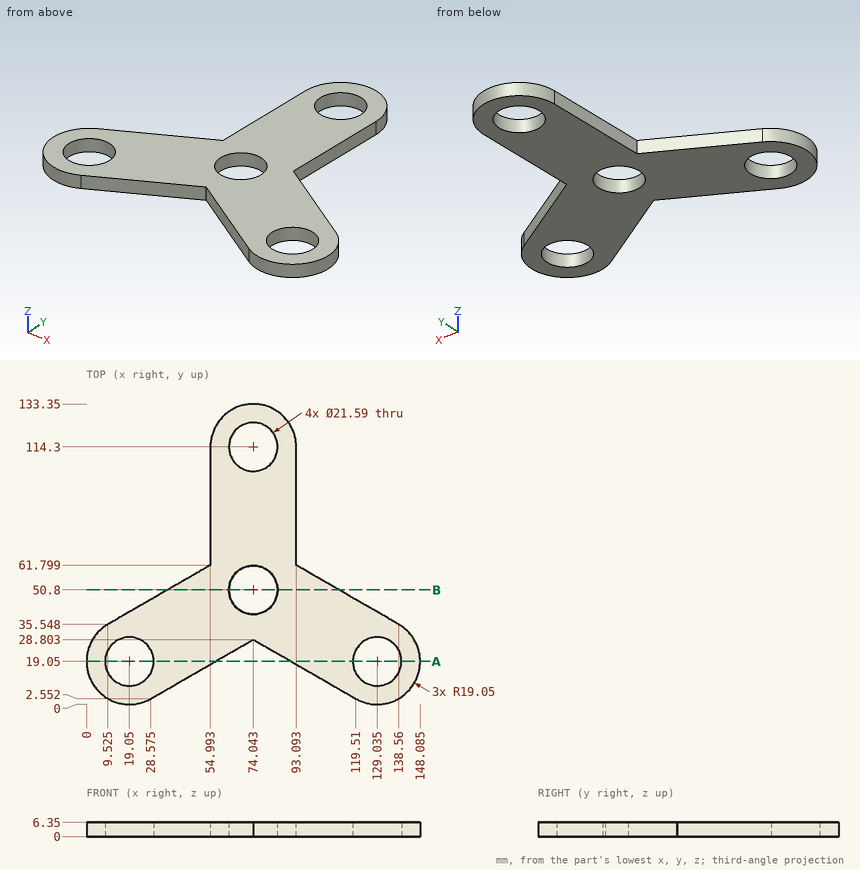
Answer from the drawing. Dimensions are ordinates in mm from the lowest x, y and z of the part. Round coordinates to 2 decimals unless told otherwise and drop trailing zeros. Order: outer loops, then holes, each group sorted by start corner. A loop starts at its lowest first (then second) coordinate and runs counter-clockwise, first axis right, second up.
1) Flat-ended cylindrical pins translate along their axes: pin 1 (1.9 mm diameter, centred on y = 87.5, z = 2, fed in from +X); pin 2 (17.5 mm diameter, centred on x = 19.05, y = 19.05, fed in from -Z); pin 3 (3 mm diameter, centred on y = 78.5, z = 3.5, fed in from -X); pin 4 (3 mm diameter, centred on x = 18, z = 4.5, fed in from +Y). Find the tip coordinate at first contact, or state that the pin passes through.
2) The part is cut by section B-B on y = 50.8. Write down the section's boundary in (x, z), plus the area to 3 significant figures.
3) The part is cut by section A-A on y = 19.05. Give the number of separate pieces and of enclosed holes in the cut face.
4) Straight lines are drawn through the part: L1, parallel to Y at x = 68, z = 4.75 (1 decimal); L2, parallel to X at y = 94, z = 5; L3, parallel to Y at x = 19.05, z = 3.75 (1 decimal). For each, find the intervals that lie inside material, in ascending order.
Resolved:
1. pin 1: stops at x = 93.09
1. pin 2: passes through
1. pin 3: stops at x = 54.99
1. pin 4: stops at y = 41.31
2. outline: (35.94, 0) - (63.25, 0) - (63.25, 6.35) - (35.94, 6.35) - close; (84.84, 0) - (112.14, 0) - (112.14, 6.35) - (84.84, 6.35) - close
2. area: 347 mm2
3. separate pieces: 4
3. enclosed holes: 0
4. L1: y = 25.3 to 41.9, 59.7 to 105.4, 123.2 to 132.4
4. L2: x = 54.99 to 93.09
4. L3: y = 0 to 8.3, 29.8 to 41
